Check sheet for the drawn part. Datum: minimum x, y, z corner. Units: mm. Give positions to 0.01 mm unless a question says otherwise; leave off trailing zeros. Write each loop counter-clockwise with the first axis right and the second up, starting at its lowest first coordinate (ties: lowest second). Pieces come first, ordered by that corner, then holes. Notation, with made-up numbers: (73.5, 5) - (113.5, 5) arc R18 ccw to (113.5, 21) - close; hole circle Ø1 at (-0.75, 65.25). An arc over 180 degrees is marked (long way). Answer as a JSON object with one key per item and string values. Group by question number.
Item 1: Scan lines: line 1 along Z through (x, y) = (26, 25) (1 decimal); line 2 along Z through (x, y) = (3, 17) (1 decimal); line 3 along Y through (x, z) = (24, 88.5) (1 decimal). Record each from-to range of solid material in increasing order. Write a range as [from, to].
Item 2: Draft check along Y on the marked faces 1, 2, 3 and 4. Enter one of: +Y half, -Y half, draft (parallel to the pull), parting line (faces both ways), or undercut.
Item 3: Go/stop test with flat-tipped pins: pin 1 (1.5 mm diameter, centred on y = 9, z = 47, fed in from +X); pin 2 (2 mm diameter, centred on x = 21.5, y = 7, fed in from -Z) (1 decimal); pin 3 (8 mm diameter, centred on y = 19.5, z = 80.5, fed in from +X). Record where each tip stops, or that it passes through.
Item 4: Sectioned sample at C-C, the plane z = 22. Record the boundary of the cut face in (x, y).
Item 5: Sectioned sample at A-A, the plane x = 11.5. Count the separate pieces of the cut face and the enclosed holes in it, and give its area (3 significant figures).
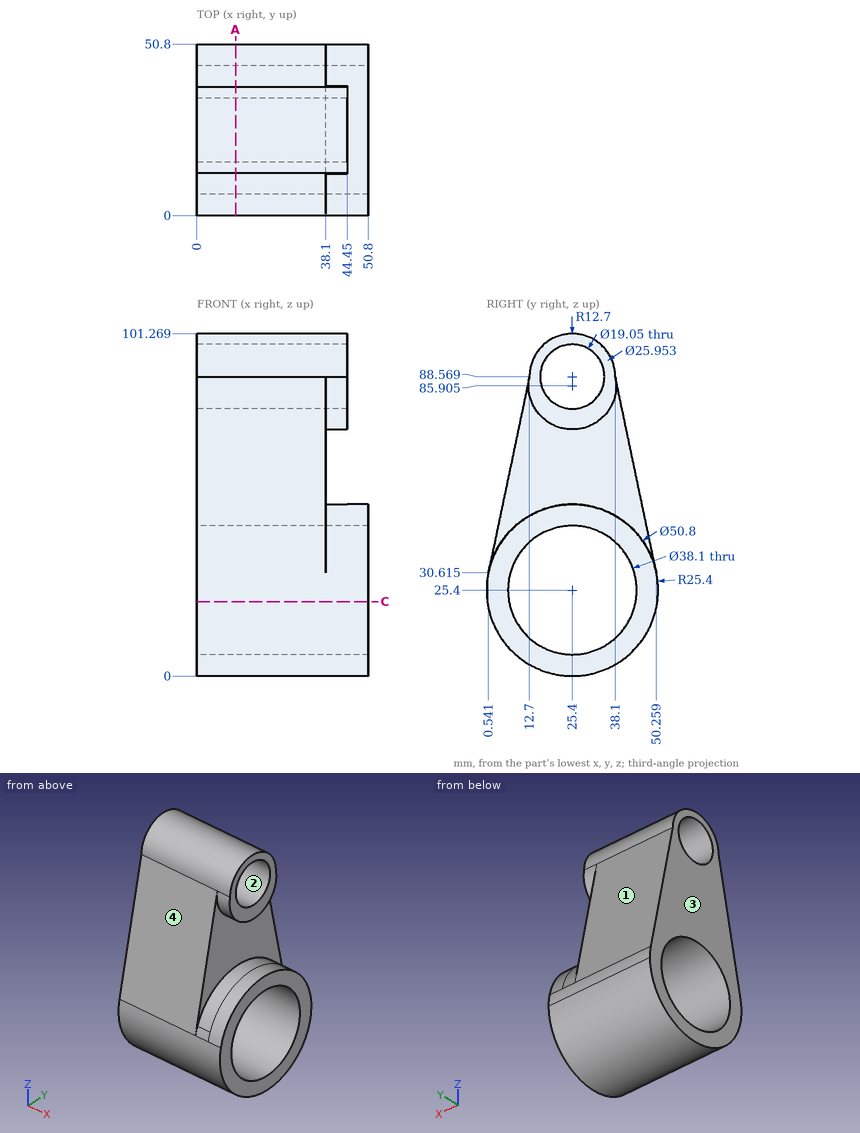
Geometry check:
{
 "1": {"line 1": "[0, 6.4], [44.4, 79.1], [98.1, 101.3]", "line 2": "[1.4, 8.3], [42.5, 84.1], [93.1, 98.1]", "line 3": "[12.7, 15.9], [34.9, 38.1]"},
 "2": {"face 1": "+Y half", "face 2": "undercut", "face 3": "draft", "face 4": "-Y half"},
 "3": {"pin 1": "x = 38.1", "pin 2": "z = 6.9", "pin 3": "x = 44.45"},
 "4": {"outline": "(0, 0.23) - (50.8, 0.23) - (50.8, 6.66) - (0, 6.66) - close; (0, 44.14) - (50.8, 44.14) - (50.8, 50.57) - (0, 50.57) - close"},
 "5": {"separate pieces": "1", "enclosed holes": "2", "area": "2,280 mm^2"}
}
